Geometry check sheet. Reference: the model listing, model coordinates, mm. Face numbers are marked on the shaded views. A direction names the side the tool comes from. Round coordinates to 2 decimals unless told otherwise and drop trailing zeros. Order: outer loops, then holes, each group sorted by start corner. A loop starts at its lowest first (then second) coordinate and runs counter-clockwise, first axis right, second up. Notation, with made-up numbers: (-22.5, 0) - (20.5, 0) arc R12 ccw to (20.5, 16) - close; hole circle Ø10 at (38, -31.75). An arc over 180 degrees is marked (long way). Return JSON: item names as keys, results as strings. Group by question number.
Q1. Gauge pin test, flat end, axial feed: pin 1 Ø16.5 at (x, z) = (0, 0) entering from +Y. Record the tip position at first contact, or that the pin passes through.
Q2. Sectioned sample at C-C, the plane z = -12. Record the cut outline in (x, y), then the cut area to 3 significant figures.
Q3. Sectioned sample at A-A, the plane y = 2.5. Give the number of separate pieces and of enclosed holes in the cut face, then the cut area to 3 significant figures.
Q4. Material ranges on line 1 along X through (y, z) = (-2.25, 0); line 2 along X through (y, z) = (-0.4, -6), recorded low to high.
Q5. Draft check along Z on the marked faces 1, 2 and 3. Enter one of: pulls with the +Z half, pulls with the -Z half, needs draft (parallel to the pull), parting line crosses it, or undercut.
Q6. Sectioned sample at B-B, the plane x = -11. Record the cut outline in (y, z), then the cut area to 3 significant figures.
Q7. Tool access check on the marked faces 4 and 5. Record the directions out of +Z, -Z, +X, -X, +Y, -Y that give a thin tool (end or side, any length) a straight path to the whole face; none if there is none.
```python
from build123d import *
from build123d.topology import SkipClean

# Parameters (mm, degrees)
SKETCH1_W           = 40
SKETCH1_H           = 40
BOSS_EXTRUDE1_DEPTH = 1
BOSS_EXTRUDE2_START = 2
SKETCH2_W           = 40
SKETCH2_H           = 40
SKETCH2_R           = 13.606270174
BOSS_EXTRUDE2_DEPTH = 2
SKETCH3_W           = 40
SKETCH3_H           = 40
SKETCH3_R           = 13.606270174
BOSS_EXTRUDE3_DEPTH = 2
CUT_EXTRUDE1_DEPTH  = 6


with BuildPart() as part:
    # Sketch1 → Boss-Extrude1 (new, symmetric)
    with BuildSketch(Plane(origin=(0, 0, 0), x_dir=(1, 0, 0), z_dir=(0, 1, 0))):
        Rectangle(SKETCH1_W, SKETCH1_H)
        with BuildLine():
            Line((-1, -1), (-1, -13.569472652))
            ThreePointArc((-1, -13.569472652), (-9.621085907, -9.621085907), (-13.569472652, -1))
            Line((-13.569472652, -1), (-1, -1))
        make_face(mode=Mode.SUBTRACT)
        with BuildLine():
            ThreePointArc((13.569472652, -1), (9.621085907, -9.621085907), (1, -13.569472652))
            Line((1, -13.569472652), (1, -1))
            Line((1, -1), (13.569472652, -1))
        make_face(mode=Mode.SUBTRACT)
        with BuildLine():
            Line((-1, 1), (-13.569472652, 1))
            ThreePointArc((-13.569472652, 1), (-9.621085907, 9.621085907), (-1, 13.569472652))
            Line((-1, 13.569472652), (-1, 1))
        make_face(mode=Mode.SUBTRACT)
        with BuildLine():
            Line((13.569472652, 1), (1, 1))
            Line((1, 1), (1, 13.569472652))
            ThreePointArc((1, 13.569472652), (9.621085907, 9.621085907), (13.569472652, 1))
        make_face(mode=Mode.SUBTRACT)
    extrude(amount=BOSS_EXTRUDE1_DEPTH, both=True)

    # Sketch2 → Boss-Extrude2 (add)
    with BuildSketch(Plane(origin=(0, 1, 0), x_dir=(1, 0, 0), z_dir=(0, 1, 0)).offset(BOSS_EXTRUDE2_START)):
        Rectangle(SKETCH2_W, SKETCH2_H)
        with Locations(Location((0, 0, 0), (0, 0, 85.785216229))):
            Circle(SKETCH2_R, mode=Mode.SUBTRACT)
    extrude(amount=-BOSS_EXTRUDE2_DEPTH)

    # Sketch3 → Boss-Extrude3 (add)
    with SkipClean():  # the faces are left unmerged after this step: merging them gives an invalid solid
        with BuildSketch(Plane.XZ.offset(1)):
            Rectangle(SKETCH3_W, SKETCH3_H)
            with Locations(Location((0, 0, 0), (0, 0, 270))):
                Circle(SKETCH3_R, mode=Mode.SUBTRACT)
        extrude(amount=BOSS_EXTRUDE3_DEPTH)

    # Sketch4 → Cut-Extrude1 (cut)
    with SkipClean():  # the faces are left unmerged after this step: merging them gives an invalid solid
        with BuildSketch(Plane(origin=(0, 3, 0), x_dir=(1, 0, 0), z_dir=(0, 1, 0))):
            with BuildLine():
                Line((-18.578772203, 17.578772203), (-18.578772203, 9.684451785))
                ThreePointArc((-18.578772203, 9.684451785), (-17.961455635, 8.760572252), (-16.871665421, 8.977345004))
                Line((-16.871665421, 8.977345004), (-8.977345004, 16.871665421))
                ThreePointArc((-8.977345004, 16.871665421), (-8.760572252, 17.961455635), (-9.684451785, 18.578772203))
                Line((-9.684451785, 18.578772203), (-17.578772203, 18.578772203))
                ThreePointArc((-17.578772203, 18.578772203), (-18.285878984, 18.285878984), (-18.578772203, 17.578772203))
            make_face()
            with BuildLine():
                Line((8.977345004, 16.871665421), (16.871665421, 8.977345004))
                ThreePointArc((16.871665421, 8.977345004), (17.961455635, 8.760572252), (18.578772203, 9.684451785))
                Line((18.578772203, 9.684451785), (18.578772203, 17.578772203))
                ThreePointArc((18.578772203, 17.578772203), (18.285878984, 18.285878984), (17.578772203, 18.578772203))
                Line((17.578772203, 18.578772203), (9.684451785, 18.578772203))
                ThreePointArc((9.684451785, 18.578772203), (8.760572252, 17.961455635), (8.977345004, 16.871665421))
            make_face()
            with BuildLine():
                Line((16.871665421, -8.977345004), (8.977345004, -16.871665421))
                ThreePointArc((8.977345004, -16.871665421), (8.760572252, -17.961455635), (9.684451785, -18.578772203))
                Line((9.684451785, -18.578772203), (17.578772203, -18.578772203))
                ThreePointArc((17.578772203, -18.578772203), (18.285878984, -18.285878984), (18.578772203, -17.578772203))
                Line((18.578772203, -17.578772203), (18.578772203, -9.684451785))
                ThreePointArc((18.578772203, -9.684451785), (17.961455635, -8.760572252), (16.871665421, -8.977345004))
            make_face()
            with BuildLine():
                Line((-8.977345004, -16.871665421), (-16.871665421, -8.977345004))
                ThreePointArc((-16.871665421, -8.977345004), (-17.961455635, -8.760572252), (-18.578772203, -9.684451785))
                Line((-18.578772203, -9.684451785), (-18.578772203, -17.578772203))
                ThreePointArc((-18.578772203, -17.578772203), (-18.285878984, -18.285878984), (-17.578772203, -18.578772203))
                Line((-17.578772203, -18.578772203), (-9.684451785, -18.578772203))
                ThreePointArc((-9.684451785, -18.578772203), (-8.760572252, -17.961455635), (-8.977345004, -16.871665421))
            make_face()
        extrude(amount=-CUT_EXTRUDE1_DEPTH, mode=Mode.SUBTRACT)


solid = part.part
```
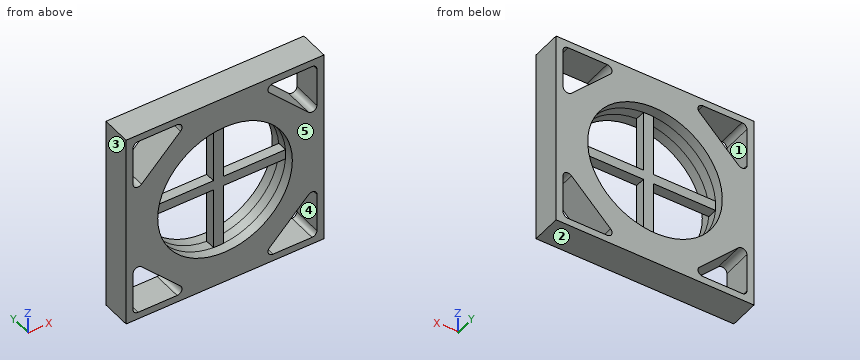
Reply:
{
 "1": {"pin 1": "y = 1"},
 "2": {"outline": "(-20, -3) - (-18.58, -3) - (-18.58, 3) - (-20, 3) - close; (-13.85, -3) - (-6.41, -3) - (-6.41, 3) - (-13.85, 3) - close; (-1, -1) - (1, -1) - (1, 1) - (-1, 1) - close; (6.41, -3) - (13.85, -3) - (13.85, 3) - (6.41, 3) - close; (18.58, -3) - (20, -3) - (20, 3) - (18.58, 3) - close", "area": "110 mm^2"},
 "3": {"separate pieces": "1", "enclosed holes": "5", "area": "773 mm^2"},
 "4": {"line 1": "-20 to -13.61, 13.61 to 20", "line 2": "-20 to -12.21, -1 to 1, 12.21 to 20"},
 "5": {"face 1": "undercut", "face 2": "pulls with the -Z half", "face 3": "needs draft"},
 "6": {"outline": "(-3, -20) - (3, -20) - (3, -18.58) - (-3, -18.58) - close; (-3, -14.85) - (3, -14.85) - (3, -8.01) - (-3, -8.01) - close; (-3, 8.01) - (3, 8.01) - (3, 14.85) - (-3, 14.85) - close; (-3, 18.58) - (3, 18.58) - (3, 20) - (-3, 20) - close; (-1, -1) - (1, -1) - (1, 1) - (-1, 1) - close", "area": "103 mm^2"},
 "7": {"face 4": "+Y, -Y", "face 5": "+Z, -Z, +X, -X, -Y"}
}
